Source: CAD feature listing. Evaluate the final solid. Frame: model axes, mm. A direction names the side the tool comes from. Round coordinates to 2 decimals unless told otherwise and drop trailing zeros. Order: outer loops, then holes, each group sorted by start corner. A loop starts at its lowest first (then second) coordinate and runs counter-clockwise, first axis right, second up. Notation, with made-up numbers: (26, 43) -> (82, 43) arc R29 cw to (82, 65) -> close; hole circle Ø3 at (-21, 66.25). An arc over 180 degrees is marked (long way). One line per item, written item: value. Start each with the question number.
1) Section A-A (x = -2.5). Return the cut outline in (y, z).
2) Reachability of faces 1 (the face through (0, 3, 13)), 2 (the face through (16.733, 3.131, 29.13)), 3 (the face through (-18, 0, 60)), 4 (the face through (-12.29, 3.13, 36.42)), 5 (the face through (19.05, 3, 17)) from +Z, -Z, +X, -X, +Y, -Y: full face, straight path, thin tool, end or side. Return the list, or none.
3) Section D-D (y = 2.25). State how many separate pieces and enclosed holes the cut face has, and give its area (3 significant figures).
4) Ray query, L1, parallel to Z at x = -11.5, y = 1.25; L2, parallel to Z at x = 14, y = 1.75; L3, parallel to Z at x = 11.5, y = 4. Return the intervals inside material, ascending.
5) Pin query (flat end, axial travel): P1, Ø3, axis at x = -3.5, y = 3.5, coming from the +Z side; P2, Ø1, axis at y = 3.5, z = 104.5, coming from the +X side; P3, Ø3, axis at x = -12.38, z = 38.42, coming from the -Y side; P4, Ø3, axis at y = 3, z = 14.5, coming from the -X side. Return the tip coordinate at first contact, or that it passes through.
6) Section C-C (z = 114.3). Return the cut outline in (x, y).
7) Section B-B (x = -17). Return the cut outline in (y, z), and give its area (3 significant figures).
```python
from build123d import *

# Parameters (mm, degrees)
SKETCH1_R           = 3
SKETCH1_R_2         = 2
BOSS_EXTRUDE1_DEPTH = 6.35
FILLET1_R           = 10.16
CUT_EXTRUDE1_DEPTH  = 125.919203888


with BuildPart() as part:
    # Sketch1 → Boss-Extrude1 (new body)
    with BuildSketch(Plane(origin=(0, 0, 0), x_dir=(1, 0, 0), z_dir=(0, 1, 0))):
        with BuildLine():
            Line((19.05, 0), (0, 0))
            Line((0, 0), (0, -22.757139607))
            ThreePointArc((0, -22.757139607), (-30.814603217, -79.553676933), (19.05, -120.65))
            ThreePointArc((19.05, -120.65), (25.4, -114.3), (19.05, -107.95))
            ThreePointArc((19.05, -107.95), (-19.05, -69.85), (19.05, -31.75))
            Line((19.05, -31.75), (19.05, 0))
        make_face()
        with Locations(Location((9.525, -9.525, 0), (0, 0, 270))):
            Circle(SKETCH1_R, mode=Mode.SUBTRACT)
        with Locations(Location((-12.380896424, -38.419103576, 0), (0, 0, 270))):
            Circle(SKETCH1_R_2, mode=Mode.SUBTRACT)
        with Locations(Location((-12.380896424, -101.280896424, 0), (0, 0, 270))):
            Circle(SKETCH1_R_2, mode=Mode.SUBTRACT)
    extrude(amount=BOSS_EXTRUDE1_DEPTH)

    # Fillet1
    # the kernel refuses this fillet: 10.16 mm, written as the material it adds along each edge
    with BuildSketch(Plane(origin=(0, 0, 22.757139607), x_dir=(0, 0, -1), z_dir=(0, 1, 0))) as fillet1_piece_1:
        with BuildLine():
            CenterArc((6.413190667, 10.16), FILLET1_R, 208.630989837, 61.369010163)
            ThreePointArc((-2.50448451, 5.291666667), (-1.175949507, 2.681941807), (0, 0))
            Line((0, 0), (6.413190667, 0))
        make_face()
    extrude(amount=6.35)
    # the kernel refuses this fillet: 10.16 mm, written as the material it takes off along each edge
    with BuildSketch(Plane(origin=(19.05, -22.696015193, 31.75), x_dir=(0, 0, -1), z_dir=(0, 1, 0))) as fillet1_2_piece_1:
        with BuildLine():
            CenterArc((9.078406077, 10.16), FILLET1_R, 192.153197469, 77.846802531)
            ThreePointArc((-0.853889939, 8.021052632), (-0.214073897, 4.033187739), (0, 0))
            Line((0, 0), (9.078406077, 0))
        make_face()
    extrude(amount=51.742030387, mode=Mode.SUBTRACT)
    with BuildSketch(Plane(origin=(0, -25.4, 0), x_dir=(1, 0, 0), z_dir=(0, 1, 0)), Plane(origin=(19.05, -25.4, 0), x_dir=(0, 0, 1), z_dir=(0, 1, 0))) as fillet1_2_piece_2:
        with BuildLine():
            CenterArc((FILLET1_R, -FILLET1_R), FILLET1_R, 90, 90)
            Line((0, -FILLET1_R), (0, 0))
            Line((0, 0), (FILLET1_R, 0))
        make_face()
    extrude(amount=57.15, mode=Mode.SUBTRACT)

    # Sketch2 → Cut-Extrude1 (cut, through all)
    with BuildSketch(Plane(origin=(0, 6.35, 0), x_dir=(1, 0, 0), z_dir=(0, 1, 0))):
        with BuildLine():
            Line((9.525, -3.255), (10.629314157, -4.648475598))
            ThreePointArc((10.629314157, -4.648475598), (10.819095226, -4.695370869), (11.006898087, -4.749648907))
            Line((11.006898087, -4.749648907), (12.66, -4.095020718))
            Line((12.66, -4.095020718), (12.919626315, -5.853963064))
            ThreePointArc((12.919626315, -5.853963064), (13.060533906, -5.989466094), (13.196036936, -6.130373685))
            Line((13.196036936, -6.130373685), (14.954979282, -6.39))
            Line((14.954979282, -6.39), (14.300351093, -8.043101913))
            ThreePointArc((14.300351093, -8.043101913), (14.354629131, -8.230904774), (14.401524402, -8.420685843))
            Line((14.401524402, -8.420685843), (15.795, -9.525))
            Line((15.795, -9.525), (14.401524402, -10.629314157))
            ThreePointArc((14.401524402, -10.629314157), (14.354629131, -10.819095226), (14.300351093, -11.006898087))
            Line((14.300351093, -11.006898087), (14.954979282, -12.66))
            Line((14.954979282, -12.66), (13.196036936, -12.919626315))
            ThreePointArc((13.196036936, -12.919626315), (13.060533906, -13.060533906), (12.919626315, -13.196036936))
            Line((12.919626315, -13.196036936), (12.66, -14.954979282))
            Line((12.66, -14.954979282), (11.006898087, -14.300351093))
            ThreePointArc((11.006898087, -14.300351093), (10.819095226, -14.354629131), (10.629314157, -14.401524402))
            Line((10.629314157, -14.401524402), (9.525, -15.795))
            Line((9.525, -15.795), (8.420685843, -14.401524402))
            ThreePointArc((8.420685843, -14.401524402), (8.230904774, -14.354629131), (8.043101913, -14.300351093))
            Line((8.043101913, -14.300351093), (6.39, -14.954979282))
            Line((6.39, -14.954979282), (6.130373685, -13.196036936))
            ThreePointArc((6.130373685, -13.196036936), (5.989466094, -13.060533906), (5.853963064, -12.919626315))
            Line((5.853963064, -12.919626315), (4.095020718, -12.66))
            Line((4.095020718, -12.66), (4.749648907, -11.006898087))
            ThreePointArc((4.749648907, -11.006898087), (4.695370869, -10.819095226), (4.648475598, -10.629314157))
            Line((4.648475598, -10.629314157), (3.255, -9.525))
            Line((3.255, -9.525), (4.648475598, -8.420685843))
            ThreePointArc((4.648475598, -8.420685843), (4.695370869, -8.230904774), (4.749648907, -8.043101913))
            Line((4.749648907, -8.043101913), (4.095020718, -6.39))
            Line((4.095020718, -6.39), (5.853963064, -6.130373685))
            ThreePointArc((5.853963064, -6.130373685), (5.989466094, -5.989466094), (6.130373685, -5.853963064))
            Line((6.130373685, -5.853963064), (6.39, -4.095020718))
            Line((6.39, -4.095020718), (8.043101913, -4.749648907))
            ThreePointArc((8.043101913, -4.749648907), (8.230904774, -4.695370869), (8.420685843, -4.648475598))
            Line((8.420685843, -4.648475598), (9.525, -3.255))
        make_face()
    extrude(amount=-CUT_EXTRUDE1_DEPTH, mode=Mode.SUBTRACT)


solid = part.part
```
Findings:
1. outline: (0, 23.02) -> (6.35, 23.02) -> (6.35, 38.43) -> (0, 38.43) -> close; (0, 101.27) -> (6.35, 101.27) -> (6.35, 115.85) -> (0, 115.85) -> close
2. face 1: -Z, -X, +Y, -Y
2. face 2: +X, +Y, -Y
2. face 3: +Z, -Z, +X, -X, -Y
2. face 4: +Y, -Y
2. face 5: -Z, +X, +Y, -Y
3. separate pieces: 1
3. enclosed holes: 3
3. area: 2,050 mm2
4. L1: 29.26 to 36.62, 40.21 to 47.08, 92.62 to 99.49, 103.08 to 110.44
4. L2: 1.38 to 6.25, 12.8 to 31.45, 107.61 to 120.4
4. L3: 0.34 to 4.55, 14.5 to 32.49, 107.19 to 120.09
5. P1: z = 116.08
5. P2: x = 4.35
5. P3: through
5. P4: x = 0
6. outline: (-5.54, 0) -> (25.4, 0) -> (25.4, 6.35) -> (-5.54, 6.35) -> close
7. outline: (0, 34.06) -> (6.35, 34.06) -> (6.35, 57.52) -> (0, 57.52) -> close; (0, 82.18) -> (6.35, 82.18) -> (6.35, 105.64) -> (0, 105.64) -> close
7. area: 298 mm2
